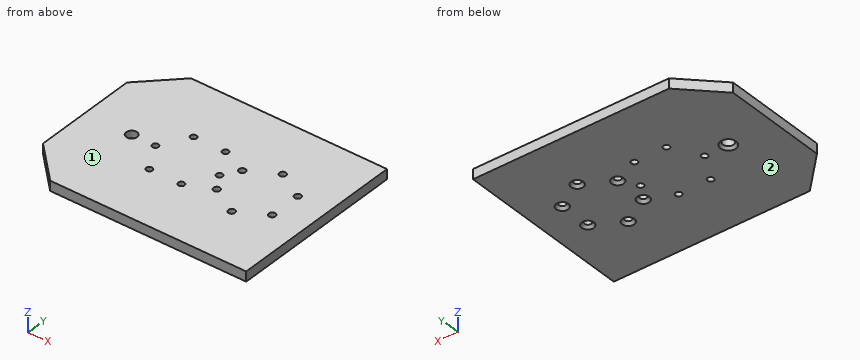
from build123d import *

# Parameters (mm, degrees)
F1_DEPTH       = 6.35
F2_D           = 7
F2_CSINK_D     = 10
F2_CSINK_ANGLE = 82
F3_D           = 4.3
F3_CSINK_D     = 7.75
F3_CSINK_ANGLE = 90
F4_D           = 4


with BuildPart() as f1:
    # F0 (on Top) → F1 (new body)
    with BuildSketch(Plane.XY):
        Polygon((-149.4, 23), (-126.4, 0), (0, 0), (0, 113.8), (-126.4, 113.8), (-149.4, 90.8), align=None)
    extrude(amount=F1_DEPTH)

    # F2 (through all)
    with Locations(Plane(origin=(0, 0, 0), x_dir=(1, 0, 0), z_dir=(0, 0, -1))):
        with Locations((-119.26, -56.9)):
            CounterSinkHole(F2_D / 2, F2_CSINK_D / 2, counter_sink_angle=F2_CSINK_ANGLE)

    # F3 (through all)
    with Locations(Plane(origin=(0, 0, 0), x_dir=(1, 0, 0), z_dir=(0, 0, -1))):
        with Locations((-38.3, -36.26), (-20.4252356659, -46.58), (-20.4252356659, -67.22), (-38.3, -77.54), (-56.1747643341, -67.22), (-56.1747643341, -46.58)):
            CounterSinkHole(F3_D / 2, F3_CSINK_D / 2, counter_sink_angle=F3_CSINK_ANGLE)

    # F4 (through all)
    with Locations(Plane(origin=(0, 0, 0), x_dir=(1, 0, 0), z_dir=(0, 0, -1))):
        with Locations((-103.94, -56.9), (-93.62, -39.0252356659), (-72.98, -39.0252356659), (-62.66, -56.9), (-72.98, -74.7747643341), (-93.62, -74.7747643341)):
            Hole(F4_D / 2)


solid = f1.part
The listing builds one solid part. Answer for the finished solid, in the listing's coordinates (mm). Face numbers are marked on the shaded views. Round coordinates to 2 decimals unless told otherwise and drop trailing zeros. Order: outer loops, then holes, each group sorted by start corner. A loop starts at its lowest first (then second) coordinate and runs counter-clockwise, first axis right, second up. Notation, with made-up numbers: M 42,58 L 61,58 A10 ccw 61,71 Z; hole C 75,-14 d11. An arc over 180 degrees is marked long. Answer in a Markdown table with one row per item. Add a question column.
1) Consider line 1 along Y through (x, z) = (-72.98, 4.5); line 2 along X through (y, z) = (46.58, 3.8); line 3 along X through (y, z) = (36.26, 2.8). Determine where each line is inside the solid, lowest interval first. Write a range as from..to.
2) Flat-ended cylindrical pins translate along their axes: pin 1 Ø3.5 at (x, y) = (-72.98, 74.77) entering from -Z; pin 2 Ø5 at (x, y) = (-20.43, 67.22) entering from -Z; pin 3 Ø7 at (x, y) = (-38.3, 77.54) entering from -Z (3 decimals). Find the tip coordinate at first contact, or state that the pin passes through.
3) The part is cut by section A-A on x = -72.98. Determine the outline of the cut face in (y, z), plus the area to 3 significant figures.
4) The part is cut by section C-C on y = 56.9. Determine the outline of the cut face in (x, z), plus the area to 3 significant figures.
5) Determine the mould class of the marked faces 1 and 2 for opening direction Z: pulls with the +Z half, pulls with the -Z half, needs draft (parallel to the pull), parting line crosses it, or undercut.
6) The part is cut by section B-B on x = -103.94. Determine the outline of the cut face in (y, z), plus the area to 3 significant figures.
7) The part is cut by section D-D on z = 4.75. Count the separate pieces of the cut face and the enclosed holes in it, plus the area to 3 significant figures.
Findings below:
| question | item | result |
|---|---|---|
| 1 | line 1 | y = 0..37.03, 41.03..72.77, 76.77..113.8 |
| 1 | line 2 | x = -149.4..-58.32, -54.02..-22.58, -18.28..0 |
| 1 | line 3 | x = -149.4..-40.45, -36.15..0 |
| 2 | pin 1 | passes through |
| 2 | pin 2 | stops at z = 1.37 |
| 2 | pin 3 | stops at z = 0.375 |
| 3 | outline | M 0,0 L 37.03,0 L 37.03,6.35 L 0,6.35 Z; M 41.03,0 L 72.77,0 L 72.77,6.35 L 41.03,6.35 Z; M 76.77,0 L 113.8,0 L 113.8,6.35 L 76.77,6.35 Z |
| 3 | area | 672 mm² |
| 4 | outline | M -149.4,0 L -124.26,0 L -122.76,1.73 L -122.76,6.35 L -149.4,6.35 Z; M -115.76,1.73 L -114.26,0 L -105.94,0 L -105.94,6.35 L -115.76,6.35 Z; M -101.94,0 L -64.66,0 L -64.66,6.35 L -101.94,6.35 Z; M -60.66,0 L 0,0 L 0,6.35 L -60.66,6.35 Z |
| 4 | area | 851 mm² |
| 5 | face 1 | pulls with the +Z half |
| 5 | face 2 | pulls with the -Z half |
| 6 | outline | M 0,0 L 54.9,0 L 54.9,6.35 L 0,6.35 Z; M 58.9,0 L 113.8,0 L 113.8,6.35 L 58.9,6.35 Z |
| 6 | area | 697 mm² |
| 7 | separate pieces | 1 |
| 7 | enclosed holes | 13 |
| 7 | area | 16,300 mm² |
